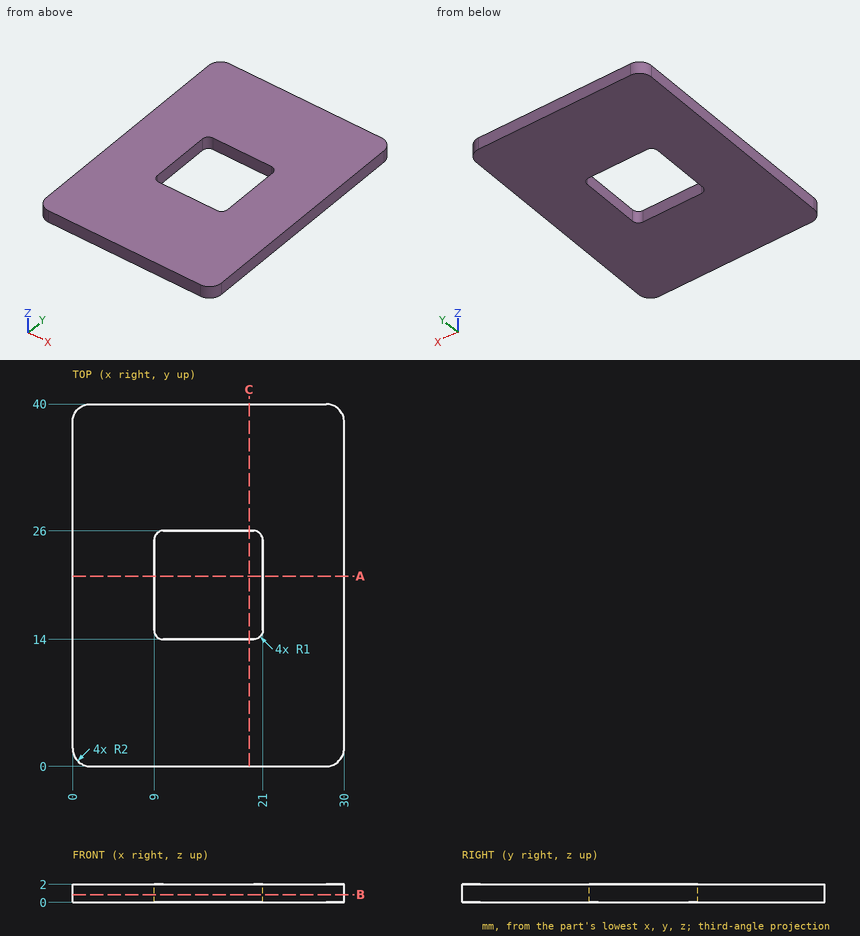
Geometry: see drawing. Coordinates: mm, zero at the bounding-box minimum. Coordinates: 2 decimals unless noted, no trailing zeros. Loops run counter-clockwise (first coordinate to the right, second up) from the corner with the lowest first, then second, coordinate; pieces in that order, holes last. Notation, with made-up numbers: (45, -37.5) - (58, -37.5) arc R16 ccw to (58, -32.5) - close; hole circle Ø2 at (-4, 5.25). An arc over 180 degrees is marked (long way). Put each result on its own line as item: value. Start each with the question number.
Q1. Cut plane A-A, the plane y = 21. Return loops of the section in (x, z), and give its area (3 significant figures).
Q2. Cut plane B-B, the plane z = 0.85. Return loops of the section in (x, y).
Q3. Line query: line 1 (X direction, y = 19, z = 0.7); line 2 (Y direction, x = 11.5, z = 1.4); line 3 (Y direction, x = 20.5, z = 1.1). Output: solid intervals per line, ascending.
Q4. Cut plane C-C, the plane x = 19.5. Return loops of the section in (y, z), and give its area (3 significant figures).
Filled sheet:
1. outline: (0, 0) - (9, 0) - (9, 2) - (0, 2) - close; (21, 0) - (30, 0) - (30, 2) - (21, 2) - close
1. area: 36.0 mm²
2. outline: (0, 2) arc R2 ccw to (2, 0) - (28, 0) arc R2 ccw to (30, 2) - (30, 38) arc R2 ccw to (28, 40) - (2, 40) arc R2 ccw to (0, 38) - close; hole (9, 15) arc R1 ccw to (10, 14) - (20, 14) arc R1 ccw to (21, 15) - (21, 25) arc R1 ccw to (20, 26) - (10, 26) arc R1 ccw to (9, 25) - close
3. line 1: 0 to 9, 21 to 30
3. line 2: 0 to 14, 26 to 40
3. line 3: 0 to 14.13, 25.87 to 40
4. outline: (0, 0) - (14, 0) - (14, 2) - (0, 2) - close; (26, 0) - (40, 0) - (40, 2) - (26, 2) - close
4. area: 56.0 mm²
